from build123d import *

# Parameters (mm, degrees)
EXTRUDE1_DEPTH = 40
SKETCH3_R      = 5
SKETCH3_R_2    = 3
EXTRUDE2_DEPTH = 5
EXTRUDE3_START = 5
SKETCH4_R      = 4
SKETCH4_R_2    = 3
EXTRUDE3_DEPTH = 5


with BuildPart() as part:
    # Sketch2 → Extrude1 (new body)
    with BuildSketch(Plane(origin=(0, 0, 0), x_dir=(1, 0, 0), z_dir=(0, 1, 0))):
        with BuildLine():
            Line((-20, 20), (20, 20))
            Line((20, 20), (20, 1))
            Line((20, 1), (11.456439237, 1))
            ThreePointArc((11.456439237, 1), (-11.5, 0), (11.456439237, -1))
            Line((11.456439237, -1), (20, -1))
            Line((20, -1), (20, -20))
            Line((20, -20), (-20, -20))
            Line((-20, -20), (-20, 20))
        make_face()
    extrude(amount=EXTRUDE1_DEPTH)

    # Sketch3 → Extrude2 (add)
    with BuildSketch(Plane.XY.offset(20)):
        with BuildLine():
            Line((-28, 170), (-28, 0))
            Line((-28, 0), (-12, 0))
            Line((-12, 0), (-12, 170))
            ThreePointArc((-12, 170), (-20, 178), (-28, 170))
        make_face()
        with Locations((-20, 170)):
            Circle(SKETCH3_R, mode=Mode.SUBTRACT)
        with Locations((-20, 110)):
            Circle(SKETCH3_R_2, mode=Mode.SUBTRACT)
    extrude(amount=EXTRUDE2_DEPTH)

    # Sketch4 → Extrude3 (add)
    with BuildSketch(Plane(origin=(0, 0, -20), x_dir=(-1, 0, 0), z_dir=(0, 0, -1)).offset(EXTRUDE3_START)):
        with BuildLine():
            Line((12, 0), (28, 0))
            Line((28, 0), (28, 170))
            ThreePointArc((28, 170), (20, 178), (12, 170))
            Line((12, 170), (12, 0))
        make_face()
        with Locations((20, 170)):
            Circle(SKETCH4_R, mode=Mode.SUBTRACT)
        with Locations(Location((20, 110, 0), (0, 0, 180))):
            Circle(SKETCH4_R_2, mode=Mode.SUBTRACT)
    extrude(amount=-EXTRUDE3_DEPTH)


solid = part.part
Geometry check sheet. Reference: the model listing, model coordinates, mm. A direction names the side the tool comes from. Give positions to 0.01 mm unless a question says otherwise; leave off trailing zeros. Loops run counter-clockwise (first coordinate to the right, second up) from the corner with the lowest first, then second, coordinate; pieces in that order, holes last. Notation, with made-up numbers: M 45,14.5 L 89,14.5 A27 ccw 89,38.5 Z; hole C -12,9 d11. An arc over 180 degrees is marked long. Answer as a JSON object with one key per item and string values. Group by question number.
Item 1: Sectioned sample at C-C on x = 0. Record the boundary of the cut face in (y, z), plus the area to 3 significant figures.
Item 2: Mould release check, pull along Z, two halves, no side actions. Record for faces 4 (the cylindrical face through (-22.4, 111.8, -22.5)), 5 (the flat face through (-20, 90, 25)), 6 (the flat face through (16, 20, 1)), 7 (the flat face through (-9, 40, 9)): pulls with the +Z half, pulls with the -Z half, needs draft (parallel to the pull), parting line crosses it, or undercut.
Item 3: Sectioned sample at A-A on y = 110. Record the boundary of the cut face in (x, z).
Item 4: Material ranges on L1, parallel to Y at x = -20, z = 21.5; L2, parallel to Y at x = -20, z = -22; L3, parallel to Z at x = -21, y = 119.5, recorded low to high.
Item 5: Sectioned sample at B-B on y = 58. Record the boundary of the cut face in (x, z).
Item 6: Gauge pin test, flat ends, axial feed: pin 1 (11.5 mm diameter, centred on x = -20, y = 170, fed in from +Z); pin 2 (10 mm diameter, centred on y = 79.5, z = 16, fed in from +X); pin 3 (9.5 mm diameter, centred on x = 3, y = 25, fed in from -Z); pin 4 (7 mm diameter, centred on x = 14.5, y = 21, fed in from +Z). Record the tip position at first contact, or that the pin passes through.
Item 7: Access from +Z, -Z, +X, -X, +Y, -Y to the whole of each face (thin tool, end or side, straight path). Record for faces 1 (the flat face through (-20, 20, 0)), 2 (the flat face through (-20, 90, -20)), 3 (the flat face through (4, 20, 20)).
Item 8: Sectioned sample at D-D on y = 14.5. Record the boundary of the cut face in (x, z), plus the area to 3 significant figures.
Findings below:
{
 "1": {"outline": "M 0,-20 L 40,-20 L 40,-11.5 L 0,-11.5 Z; M 0,11.5 L 40,11.5 L 40,20 L 0,20 Z", "area": "680 mm2"},
 "2": {"face 4": "needs draft", "face 5": "pulls with the +Z half", "face 6": "undercut", "face 7": "undercut"},
 "3": {"outline": "M -28,-25 L -23,-25 L -23,-20 L -28,-20 Z; M -28,20 L -23,20 L -23,25 L -28,25 Z; M -17,-25 L -12,-25 L -12,-20 L -17,-20 Z; M -17,20 L -12,20 L -12,25 L -17,25 Z"},
 "4": {"L1": "0 to 107, 113 to 165, 175 to 178", "L2": "0 to 107, 113 to 166, 174 to 178", "L3": "-25 to -20, 20 to 25"},
 "5": {"outline": "M -28,-25 L -12,-25 L -12,-20 L -28,-20 Z; M -28,20 L -12,20 L -12,25 L -28,25 Z"},
 "6": {"pin 1": "z = 25", "pin 2": "x = -12", "pin 3": "z = -20", "pin 4": "z = 20"},
 "7": {"face 1": "-X, +Y, -Y", "face 2": "-X, +Y", "face 3": "+Z, +X, +Y, -Y"},
 "8": {"outline": "M -28,-25 L -12,-25 L -12,-20 L 20,-20 L 20,-1 L 11.46,-1 A11.5 cw long 11.46,1 L 20,1 L 20,20 L -12,20 L -12,25 L -28,25 L -28,20 L -20,20 L -20,-20 L -28,-20 Z", "area": "1,330 mm2"}
}
